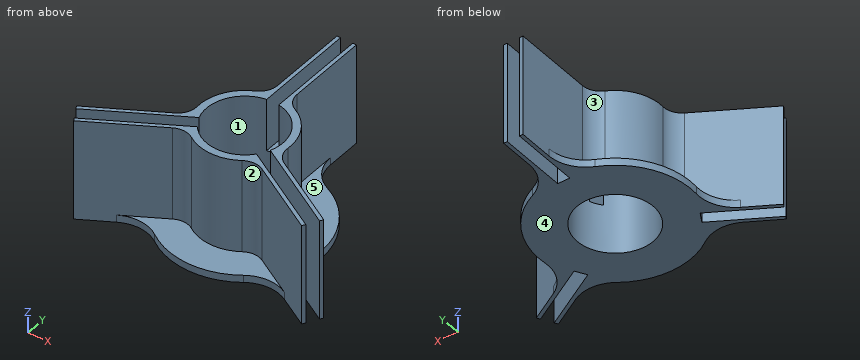
```python
from build123d import *

# Parameters (mm, degrees)
SKETCH1_R                       = 20.75
BOSS_EXTRUDE1_DEPTH             = 100
BOSS_EXTRUDE2_DEPTH             = 3.2
THICKEN1_OUTLINE_R              = 24.85
THICKEN1_OUTLINE_R_2            = 20.85
THICKEN1_DEPTH                  = 100
THICKEN2_START                  = 26.35
THICKEN2_DEPTH                  = 73.65
THICKEN2_2_OUTLINE_W            = 2
THICKEN2_2_OUTLINE_H            = 37
THICKEN2_2_DEPTH                = 26.35
THICKEN3_START                  = 26.35
THICKEN3_DEPTH                  = 73.65
THICKEN3_2_OUTLINE_W            = 2
THICKEN3_2_OUTLINE_H            = 37
THICKEN3_2_DEPTH                = 26.35
BOSS_EXTRUDE4_REACH             = 129.446
SKETCH4_W                       = 26.35
SKETCH4_H                       = 17.15
BOSS_EXTRUDE4_DIRECTION_2_REACH = 129.446
FILLET1_R                       = 10
SKETCH3_R                       = 41.5
BOSS_EXTRUDE3_DEPTH             = 4
FILLET2_R                       = 20
CIRPATTERN4_COUNT               = 3
MOVE_FACE3_BY                   = 0.1
MOVE_FACE4_BY                   = 0.1
MOVE_FACE4_2_BY                 = 0.1
MOVE_FACE4_3_BY                 = 0.1
MOVE_START                      = 26.35
MOVE_FACE5_OUTLINE_W            = 6.6
MOVE_FACE5_OUTLINE_H            = 20.75
MOVE_FACE5_DEPTH                = 73.65
CIRPATTERN1_COUNT               = 3
SKETCH5_R                       = 108.755446709
CUT_EXTRUDE1_DEPTH              = 45


with BuildPart() as part:
    # Sketch1 → Boss-Extrude1 (new body)
    with BuildSketch(Plane.XY):
        Circle(SKETCH1_R)
    extrude(amount=BOSS_EXTRUDE1_DEPTH)

    # Move Face3: a curved face moved outward by 0.1
    add(Solid.thicken(part.faces().sort_by_distance((-20.75, 0, 50))[0], MOVE_FACE3_BY))


with BuildPart() as body_2:
    # Sketch2 → Boss-Extrude2 (new, symmetric)
    with BuildSketch(Plane(origin=(0, 0, 0), x_dir=(0, 0, -1), z_dir=(1, 0, 0))):
        Polygon((-26.35, 20.75), (-26.35, 38), (0, 38), (0, 75), (-100, 75), (-100, 20.75), align=None)
    extrude(amount=BOSS_EXTRUDE2_DEPTH, both=True)

    # Move Face4: a face moved outward by 0.1
    extrude(body_2.faces().sort_by_distance((0, 38, 13.175))[0], amount=MOVE_FACE4_BY, dir=(0, -1, 0))

    # Move Face4 2: a face moved outward by 0.1
    extrude(body_2.faces().sort_by_distance((-3.2, 49.566782958, 53.367562563))[0], amount=MOVE_FACE4_2_BY, dir=(-1, 0, 0))

    # Move Face4 3: a face moved outward by 0.1
    extrude(body_2.faces().sort_by_distance((3.2, 49.566782958, 53.367562563))[0], amount=MOVE_FACE4_3_BY, dir=(1, 0, 0))

    # Move Face5: read off the stored shape, not the designer's step
    # Move Face5 outline → Move Face5 (add)
    with BuildSketch(Plane.XY.offset(MOVE_START)):
        with Locations((0, 10.375)):
            Rectangle(MOVE_FACE5_OUTLINE_W, MOVE_FACE5_OUTLINE_H)
    extrude(amount=MOVE_FACE5_DEPTH)


with BuildPart() as body_3:
    # Thicken1: read off the stored shape, not the designer's step
    # Thicken1 outline → Thicken1 (new body)
    with BuildSketch(Plane.XY):
        Circle(THICKEN1_OUTLINE_R)
        Circle(THICKEN1_OUTLINE_R_2, mode=Mode.SUBTRACT)
    extrude(amount=THICKEN1_DEPTH)

    # Thicken2: read off the stored shape, not the designer's step
    # Thicken2 outline → Thicken2 (add)
    with BuildSketch(Plane.XY.offset(THICKEN2_START)):
        with BuildLine():
            ThreePointArc((-5.3, 24.27823099), (-4.303593806, 24.474508787), (-3.3, 24.629910678))
            Line((-3.3, 24.629910678), (-3.3, 75))
            Line((-3.3, 75), (-5.3, 75))
            Line((-5.3, 75), (-5.3, 24.27823099))
        make_face()
    extrude(amount=THICKEN2_DEPTH)

    # Thicken2 2 outline → Thicken2 2 (add)
    with BuildSketch(Plane.XY):
        with Locations((-4.3, 56.5)):
            Rectangle(THICKEN2_2_OUTLINE_W, THICKEN2_2_OUTLINE_H)
    extrude(amount=THICKEN2_2_DEPTH)

    # Thicken3: read off the stored shape, not the designer's step
    # Thicken3 outline → Thicken3 (add)
    with BuildSketch(Plane.XY.offset(THICKEN3_START)):
        with BuildLine():
            Line((3.3, 75), (3.3, 24.629910678))
            ThreePointArc((3.3, 24.629910678), (4.303593806, 24.474508787), (5.3, 24.27823099))
            Line((5.3, 24.27823099), (5.3, 75))
            Line((5.3, 75), (3.3, 75))
        make_face()
    extrude(amount=THICKEN3_DEPTH)

    # Thicken3 2 outline → Thicken3 2 (add)
    with BuildSketch(Plane.XY):
        with Locations((4.3, 56.5)):
            Rectangle(THICKEN3_2_OUTLINE_W, THICKEN3_2_OUTLINE_H)
    extrude(amount=THICKEN3_2_DEPTH)

    # Boss-Extrude4: up to this face of the body (flat: up to its plane)
    boss_extrude4_end = Plane(body_3.part.faces().sort_by_distance((5.3, 51.059106065, 52.826548797))[0])
    # Sketch4 → Boss-Extrude4 (add, up to the picked face)
    with BuildSketch(Plane(origin=(0, 0, 0), x_dir=(0, 0, -1), z_dir=(1, 0, 0)), mode=Mode.PRIVATE) as boss_extrude4_sk1:
        with Locations((-13.175, 29.425)):
            Rectangle(SKETCH4_W, SKETCH4_H)
    boss_extrude4_tool1 = split(extrude(boss_extrude4_sk1.sketch, amount=BOSS_EXTRUDE4_REACH, mode=Mode.PRIVATE), bisect_by=boss_extrude4_end, keep=Keep.BOTH, mode=Mode.PRIVATE)
    add(boss_extrude4_tool1.solids().sort_by(Axis((0, 29.425, 13.175), (1, 0, 0)))[0])

    # Boss-Extrude4 direction 2: up to this face of the body (flat: up to its plane)
    boss_extrude4_direction_2_end = Plane(body_3.part.faces().sort_by_distance((-5.3, 51.059106065, 52.826548797))[0])
    # Sketch4 → Boss-Extrude4 direction 2 (add, up to the picked face)
    with BuildSketch(Plane(origin=(0, 0, 0), x_dir=(0, 0, -1), z_dir=(1, 0, 0)), mode=Mode.PRIVATE) as boss_extrude4_direction_2_sk1:
        with Locations((-13.175, 29.425)):
            Rectangle(SKETCH4_W, SKETCH4_H)
    boss_extrude4_direction_2_tool1 = split(extrude(boss_extrude4_direction_2_sk1.sketch, amount=-BOSS_EXTRUDE4_DIRECTION_2_REACH, mode=Mode.PRIVATE), bisect_by=boss_extrude4_direction_2_end, keep=Keep.BOTH, mode=Mode.PRIVATE)
    add(boss_extrude4_direction_2_tool1.solids().sort_by(Axis((0, 29.425, 13.175), (-1, 0, 0)))[0])

    # Fillet1
    fillet1_edges = [body_3.edges().sort_by_distance(p)[0] for p in [
        (-5.3, 24.27823099, 50),
        (5.3, 24.27823099, 50),
    ]]
    fillet(fillet1_edges, radius=FILLET1_R)

    # Sketch3 → Boss-Extrude3 (add)
    with BuildSketch(Plane.XY):
        Circle(SKETCH3_R)
    extrude(amount=BOSS_EXTRUDE3_DEPTH)

    # Fillet2
    fillet2_edges = [body_3.edges().sort_by_distance(p)[0] for p in [
        (-5.3, 41.160174927, 2),
        (5.3, 41.160174927, 2),
    ]]
    fillet(fillet2_edges, radius=FILLET2_R)


with BuildPart() as cirpattern4_1:
    # CirPattern4: pattern copy
    add(body_3.part.rotate(Axis((0, 0, 0), (0, 0, 1)), 1 * 360 / CIRPATTERN4_COUNT))


with BuildPart() as cirpattern4_2:
    # CirPattern4: pattern copy
    add(body_3.part.rotate(Axis((0, 0, 0), (0, 0, 1)), 2 * 360 / CIRPATTERN4_COUNT))

    # Combine2: read off the stored shape, not the designer's step
    # Combine2: union CirPattern4_1, body 3
    add(cirpattern4_1.part)
    add(body_3.part)


with BuildPart() as cirpattern1_1:
    # CirPattern1: pattern copy
    add(body_2.part.rotate(Axis((0, 0, 0), (0, 0, 1)), 1 * 360 / CIRPATTERN1_COUNT))


with BuildPart() as cirpattern1_2:
    # CirPattern1: pattern copy
    add(body_2.part.rotate(Axis((0, 0, 0), (0, 0, 1)), 2 * 360 / CIRPATTERN1_COUNT))


with BuildPart() as cirpattern4_2_1:
    add(cirpattern4_2.part)

    # Combine3: read off the stored shape, not the designer's step
    # Combine3: cut CirPattern1_2, CirPattern1_1, body 2, part
    add(cirpattern1_2.part, mode=Mode.SUBTRACT)
    add(cirpattern1_1.part, mode=Mode.SUBTRACT)
    add(body_2.part, mode=Mode.SUBTRACT)
    add(part.part, mode=Mode.SUBTRACT)

    # Sketch5 → Cut-Extrude1 (cut)
    with BuildSketch(Plane.XY.offset(100)):
        Circle(SKETCH5_R)
    extrude(amount=-CUT_EXTRUDE1_DEPTH, mode=Mode.SUBTRACT)


solid = cirpattern4_2_1.part
```
CAD build for the part. Positions are in the model's coordinates, mm. Face numbers are marked on the shaded views. A direction names the side the tool comes from. Round coordinates to 2 decimals unless told otherwise and drop trailing zeros. Order: outer loops, then holes, each group sorted by start corner. A loop starts at its lowest first (then second) coordinate and runs counter-clockwise, first axis right, second up.
Q1. Slice it at B-B (y = 47). Write the cut outline in (x, z).
Q2. Slice it at A-A (x = 48). Write the cut outline in (y, z), and give its area (3 significant figures).
Q3. Slice it at D-D (y = 28.5). Write the cut outline in (x, z), and give its area (3 significant figures).
Q4. Which spindle directions (+Z, -Z, +X, -X, +Y, -Y) get a long thin tool onto all of the face, cutting with end or side? Do the marked faces 1, 2, 3, 4 and 5. Say none if no direction does.
Q5. Drop flat-ended pins along their axis: pin 1 (4 mm diameter, centred on x = 46.5, z = 40.5, fed in from +Y); pin 2 (6 mm diameter, centred on x = -37, z = 33, fed in from +Y); pin 3 (1.5 mm diameter, centred on x = -17.5, z = 34, fed in from +Y). Give the stop position or say it passes through.
Q6. Wall check: L1, parallel to X at y = 0, z = 33; L2, parallel to Y at x = 0, z = 23; L3, parallel to X at y = 37, z = 47.5. Give the ranges that are in metal, low to high.
Results below:
1. outline: (-7.47, 0) - (-3.3, 0) - (-3.3, 55) - (-5.3, 55) - (-5.3, 4) - (-7.47, 4) - close; (3.3, 0) - (7.47, 0) - (7.47, 4) - (5.3, 4) - (5.3, 55) - (3.3, 55) - close
2. outline: (-33.83, 0) - (-31.52, 0) - (-31.52, 55) - (-33.83, 55) - close; (-23.9, 0) - (-21.15, 0) - (-21.15, 4) - (-21.59, 4) - (-21.59, 55) - (-23.9, 55) - close
2. area: 256 mm2
3. outline: (-30.17, 0) - (30.17, 0) - (30.17, 4) - (5.7, 4) - (5.7, 55) - (3.3, 55) - (3.3, 26.35) - (-3.3, 26.35) - (-3.3, 55) - (-5.7, 55) - (-5.7, 4) - (-30.17, 4) - close
3. area: 634 mm2
4. face 1: +Z, -Z
4. face 2: +Z, -Y
4. face 3: +Z, -X, +Y
4. face 4: -Z, +X, -X, +Y, -Y
4. face 5: +Z, +X, +Y
5. pin 1: stops at y = -19.57
5. pin 2: stops at y = -13.51
5. pin 3: stops at y = 18.36
6. L1: x = -24.85 to -20.85, 20.85 to 24.85
6. L2: y = -24.85 to -20.85, 20.85 to 37.9
6. L3: x = -5.3 to -3.3, 3.3 to 5.3
